```python
from build123d import *

# Parameters (mm, degrees)
SKETCH2_W = 24
SKETCH2_H = 8


with BuildPart() as part:
    # Sketch1 → Revolve1 (revolve)
    with BuildSketch(Plane.XY, mode=Mode.PRIVATE) as revolve1_sk:
        Polygon((0, 0), (0, 12.5), (2, 12.5), (2, 15), (22, 15), (22, 12.5), (24, 12.5), (24, 0), align=None)
    revolve(revolve1_sk.sketch.rotate(Axis((-4.047229768, 0, 0), (1, 0, 0)), 90), axis=Axis((-4.047229768, 0, 0), (1, 0, 0)))

    # Sketch2 → Cut-Revolve1 (revolve, cut)
    with BuildSketch(Plane.XY, mode=Mode.PRIVATE) as cut_revolve1_sk:
        with Locations((12, 4)):
            Rectangle(SKETCH2_W, SKETCH2_H)
    revolve(cut_revolve1_sk.sketch.rotate(Axis((-2.968632144, 0, 0), (1, 0, 0)), 90), axis=Axis((-2.968632144, 0, 0), (1, 0, 0)), mode=Mode.SUBTRACT)


solid = part.part
```
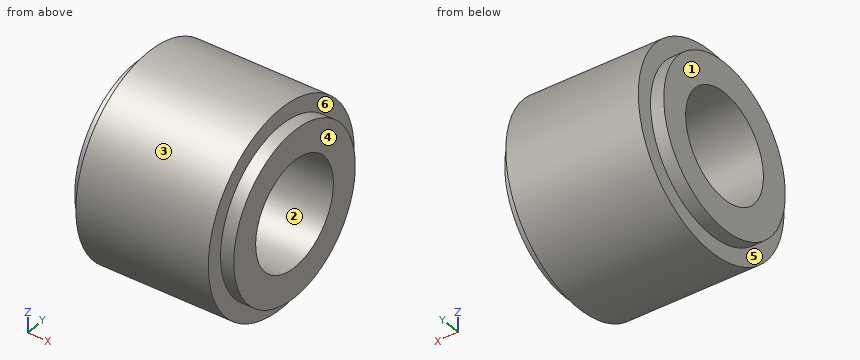
Build history of the part. All positions in model axes, mm. Face numbers are marked on the shaded views. A direction names the side the tool comes from. Coordinates: 2 decimals unless noted, no trailing zeros. Order: outer loops, then holes, each group sorted by start corner. A loop starts at its lowest first (then second) coordinate and runs counter-clockwise, first axis right, second up. Notation, with made-up numbers: (55.5, 86) -> (108.5, 86) arc R21 ccw to (108.5, 100) -> close; hole circle Ø7 at (80.5, 25). An arc over 180 degrees is marked (long way). Answer in a Markdown table with one row per item. Add a question column.
Q1. Mould opens along Z. For the marked faces 1, 2 and 3 say: +Z half, -Z half, draft (parallel to the pull), parting line (faces both ways), or undercut.
Q2. Band-saw the part on C-C, the plane x = 11.5. List the corners of the cut face in (y, z), then the cut area to 3 significant figures.
Q3. Drop flat-ended pins along their axis: pin 1 (5 mm diameter, centred on x = 14.5, z = 5.5, fed in from +Y); pin 2 (14.5 mm diameter, centred on y = 0, z = 0, fed in from -X); pin 3 (1 mm diameter, centred on x = 19.5, z = 1.5, fed in from -Y); pin 4 (1.5 mm diameter, centred on x = 15.5, z = 6, fed in from +Y). Give the stop position or say it passes through.
Q4. Band-saw the part on A-A, the plane y = 0. List the corners of the cut face in (x, z), then the cut area to 3 significant figures.
Q5. Band-saw the part on D-D, the plane z = 11.75. List the corners of the cut face in (x, y), then the cut area to 3 significant figures.
Q6. Wall check: line 1 along Y through (x, z) = (6.75, 0); line 2 along X through (y, z) = (-8, 12.5); line 3 along Z through (x, y) = (13.5, -1.25). Give the ranges that are in metal, low to high. Write a range as [from, to].
Q7. Which spindle directions (+Z, -Z, +X, -X, +Y, -Y) get a long thin tool onto all of the face, cutting with end or side? Do the marked faces 4, 5 and 6. Say none if no direction does.
Answers follow:
| question | item | result |
|---|---|---|
| 1 | face 1 | draft |
| 1 | face 2 | undercut |
| 1 | face 3 | parting line |
| 2 | outline | circle Ø30 at (0, 0); hole circle Ø16 at (0, 0) |
| 2 | area | 506 mm^2 |
| 3 | pin 1 | y = 14.7 |
| 3 | pin 2 | through |
| 3 | pin 3 | y = -14.97 |
| 3 | pin 4 | y = 14.05 |
| 4 | outline | (0, -12.5) -> (2, -12.5) -> (2, -15) -> (22, -15) -> (22, -12.5) -> (24, -12.5) -> (24, -8) -> (0, -8) -> close; (0, 8) -> (24, 8) -> (24, 12.5) -> (22, 12.5) -> (22, 15) -> (2, 15) -> (2, 12.5) -> (0, 12.5) -> close |
| 4 | area | 316 mm^2 |
| 5 | outline | (0, -4.26) -> (2, -4.26) -> (2, -9.32) -> (22, -9.32) -> (22, -4.26) -> (24, -4.26) -> (24, 4.26) -> (22, 4.26) -> (22, 9.32) -> (2, 9.32) -> (2, 4.26) -> (0, 4.26) -> close |
| 5 | area | 407 mm^2 |
| 6 | line 1 | [-15, -8], [8, 15] |
| 6 | line 2 | [2, 22] |
| 6 | line 3 | [-14.95, -7.9], [7.9, 14.95] |
| 7 | face 4 | +Z, -Z, +X, +Y, -Y |
| 7 | face 5 | -X |
| 7 | face 6 | +X |
